Autodesk Inventor part; units mm, degrees
ref_plane "YZ Plane" through (0, 0, 0) normal (1, 0, 0) x (0, 1, 0)
ref_plane "XZ Plane" through (0, 0, 0) normal (0, 1, 0) x (-1, 0, 0)
ref_plane "XY Plane" through (0, 0, 0) normal (0, 0, 1) x (1, 0, 0)
sketch "Sketch1" plane through (0, 0, 0) normal (0, 0, 1) x (1, 0, 0)
  circle A0 centre (0, 0) radius 21.15 construction
  line L0 (-18, -23) -> (18, -23) construction
  line L1 (-18, -23) -> (-18, -38.1522) construction
  line L2 (18, -23) -> (18, -38.1522) construction
  line L3 (-23, -21) -> (-23, -23)
  line L4 (-23, -23) -> (-2, -23)
  line L5 (-2, -21.0552) -> (-2, -23)
  line L6 (2, -21.0552) -> (2, -23)
  line L7 (2, -23) -> (23, -23)
  line L8 (23, -23) -> (23, -21)
  line L9 (23, -21) -> (15.5468, -21)
  line L10 (-23, -21) -> (-15.5468, -21)
  arc A1 (2, -21.0552) -> (-2, -21.0552) centre (0, 0) ccw
  arc A2 (14.2802, -17.4521) -> (15.5468, -21) centre (15.5468, -19) ccw
  arc A3 (-15.5468, -21) -> (-14.2802, -17.4521) centre (-15.5468, -19) ccw
  circle A4 centre (-24, 0) radius 2
  circle A5 centre (24, 0) radius 2
  line L11 (-22.1924, 4) -> (-24, 4)
  arc A6 (-24, 4) -> (-24, -4) centre (-24, 0) ccw
  line L12 (-24, -4) -> (-22.1924, -4)
  line L13 (22.1924, 4) -> (24, 4)
  arc A7 (24, -4) -> (24, 4) centre (24, 0) ccw
  line L14 (24, -4) -> (22.1924, -4)
  arc A8 (-22.1924, -4) -> (-14.2802, -17.4521) centre (0, 0) ccw
  arc A9 (14.2802, -17.4521) -> (22.1924, -4) centre (0, 0) ccw
  arc A10 (22.1924, 4) -> (-22.1924, 4) centre (0, 0) ccw
  point P0 (0, -23)
  point P1 (8.216, -21)
  point P2 (-8.216, -21)
  dimension "d13" = 42.3
  dimension "d1" = 23
  dimension "d2" = 36
  dimension "d3" = 2
  dimension "d5" = 5
  dimension "d6" = 2
  dimension "d7" = 4
  dimension "d14" = 4
  dimension "d15" = 4
  dimension "d16" = 48
  dimension "d17" = 24
  dimension "d18" = 4
  dimension "d19" = 22.55
extrude "Extrusion1" add sketch "Sketch1" along normal blind 10
sketch "Sketch2" plane through (2, -23, 0) normal (0, -1, 0) x (1, 0, 0)
  circle A0 centre (16, 5) radius 1.5
  line L0 (21, 0) -> (21, 10)
  point P0 (-2, 0)
  point P1 (16, 0)
  point P2 (16, 0)
  point P3 (16, 0)
  point P4 (21, 5)
  dimension "d10" = 3
extrude "Extrusion2" cut sketch "Sketch2" against normal up to surface (2 mm away)
mirror "Mirror1" about plane through (0, 0, 0) normal (1, 0, 0) of "Extrusion2"
properties part number "OmegaRing" material "ABS Plastic"
Work out the finished part from the listing and answer in its coordinate system (mm). A direction names the side the tool comes from. Give positions to 0.01 mm unless a question says otherwise; leave off trailing zeros. Write each loop counter-clockwise with the first axis right and the second up, starting at its lowest first coordinate (ties: lowest second). Pieces come first, ordered by that corner, then holes. Notation, with made-up numbers: (30.25, 36.25) - (63.25, 36.25) arc R19 cw to (63.25, 45.25) - close; hole circle Ø10 at (56, 8.5). An arc over 180 degrees is marked (long way). Use one line per item in the form item = value.
1. A cutting plane is placed at D-D (z = 1). Write down the section's boundary in (x, y), and give its area (3 significant figures).
Filled in:
outline = (-24, -4) - (-22.19, -4) arc R22.55 ccw to (-14.28, -17.45) arc R2 cw to (-15.55, -21) - (-23, -21) - (-23, -23) - (-2, -23) - (-2, -21.06) arc R21.15 cw (long way) to (2, -21.06) - (2, -23) - (23, -23) - (23, -21) - (15.55, -21) arc R2 cw to (14.28, -17.45) arc R22.55 ccw to (22.19, -4) - (24, -4) arc R4 ccw to (24, 4) - (22.19, 4) arc R22.55 ccw to (-22.19, 4) - (-24, 4) arc R4 ccw to start; hole circle Ø4 at (-24, 0); hole circle Ø4 at (24, 0)
area = 326 mm^2
2. A cutting plane is placed at B-B (y = 0). Write down the section's boundary in (x, z).
Filled in:
outline = (-28, 0) - (-26, 0) - (-26, 10) - (-28, 10) - close; (-22, 0) - (-21.15, 0) - (-21.15, 10) - (-22, 10) - close; (21.15, 0) - (22, 0) - (22, 10) - (21.15, 10) - close; (26, 0) - (28, 0) - (28, 10) - (26, 10) - close
3. Each of these flat-tipped pins is pushed along its axis until it touches: pin 1 Ø5 at (y, z) = (-16, 8.5) entering from -X; pin 2 Ø0.5 at (x, z) = (23.5, 7) entering from +Y; pin 3 Ø4 at (y, z) = (-8.5, 8) entering from +X. Where does it stop, or does it pass through?
Filled in:
pin_1 = -18.06
pin_2 = 4
pin_3 = 21.59
4. For faces 5 (the face through (23, 4, 5)), 6 (the face through (20, -21, 5)), 7 (the face through (-23, -22, 5)), determine the directions among +Z, -Z, +X, -X, +Y, -Y from which every point of the face is accessible in a straight line to the end or side of a thin tool.
Filled in:
face_5 = +Z, -Z, +X, +Y
face_6 = +Z, -Z, +X
face_7 = +Z, -Z, -X, -Y
5. A cutting plane is placed at A-A (z = 5). State how many separate pieces and enclosed holes the cut face has, and give its area (3 significant figures).
Filled in:
separate_pieces = 3
enclosed_holes = 2
area = 314 mm^2
6. A cutting plane is placed at C-C (x = -11). Write down the section's boundary in (y, z), and give its area (3 significant figures).
Filled in:
outline = (-23, 0) - (-18.06, 0) - (-18.06, 10) - (-23, 10) - close; (18.06, 0) - (19.69, 0) - (19.69, 10) - (18.06, 10) - close
area = 65.6 mm^2
7. Determine the mould class of faces 1 (the face through (13.675, -19.705, 4.93)), 2 (the face through (-13, -23, 5)), 3 (the face through (23, -22, 5)), 4 (the face through (-23, 4, 5)) for opening direction Y: released by +Y, released by -Y, zero draft, split by the parting line, or undercut.
Filled in:
face_1 = undercut
face_2 = released by -Y
face_3 = zero draft
face_4 = released by +Y
8. Consider L1, parallel to Y at x = -24, z = 6.5; L2, parallel to Z at x = 18, y = -22; L3, parallel to Y at x = 12.5, z = 2.5. Determine where each line is inside the solid, lowest interval first.
Filled in:
L1 = -4 to -2, 2 to 4
L2 = 0 to 3.5, 6.5 to 10
L3 = -23 to -17.06, 17.06 to 18.77
